```python
from build123d import *

# Parameters (mm, degrees)
SKETCH1_W           = 70
SKETCH1_H           = 70
BOSS_EXTRUDE1_DEPTH = 1
SKETCH2_R           = 25
SKETCH2_R_2         = 23
BOSS_EXTRUDE2_DEPTH = 27
SKETCH3_R           = 2.5
CUT_EXTRUDE1_DEPTH  = 1
SKETCH4_R           = 2.5
CUT_EXTRUDE2_DEPTH  = 1


with BuildPart() as part:
    # Sketch1 → Boss-Extrude1 (new body)
    with BuildSketch(Plane(origin=(0, 0, 0), x_dir=(1, 0, 0), z_dir=(0, 1, 0))):
        Rectangle(SKETCH1_W, SKETCH1_H)
    extrude(amount=BOSS_EXTRUDE1_DEPTH)

    # Sketch2 → Boss-Extrude2 (add)
    with BuildSketch(Plane.XZ):
        with Locations(Location((0, 0, 0), (0, 0, 90))):
            Circle(SKETCH2_R)
        with Locations(Location((0, 0, 0), (0, 0, 270))):
            Circle(SKETCH2_R_2, mode=Mode.SUBTRACT)
    extrude(amount=BOSS_EXTRUDE2_DEPTH)

    # Sketch3 → Cut-Extrude1 (cut)
    with BuildSketch(Plane(origin=(0, 1, 0), x_dir=(1, 0, 0), z_dir=(0, 1, 0))):
        with Locations(Location((0, 0, 0), (0, 0, 270))):
            Circle(SKETCH3_R)
        with Locations(Location((0, 17, 0), (0, 0, 270))):
            Circle(SKETCH3_R)
        with Locations(Location((17, 0, 0), (0, 0, 270))):
            Circle(SKETCH3_R)
        with Locations(Location((0, -17, 0), (0, 0, 270))):
            Circle(SKETCH3_R)
        with Locations(Location((-17, 0, 0), (0, 0, 270))):
            Circle(SKETCH3_R)
    extrude(amount=-CUT_EXTRUDE1_DEPTH, mode=Mode.SUBTRACT)

    # Sketch4 → Cut-Extrude2 (cut)
    with BuildSketch(Plane(origin=(0, 1, 0), x_dir=(1, 0, 0), z_dir=(0, 1, 0))):
        with Locations(Location((21, 21, 0), (0, 0, 270))):
            Circle(SKETCH4_R)
        with Locations(Location((21, -21, 0), (0, 0, 270))):
            Circle(SKETCH4_R)
        with Locations(Location((-21, 21, 0), (0, 0, 270))):
            Circle(SKETCH4_R)
        with Locations(Location((-21, -21, 0), (0, 0, 270))):
            Circle(SKETCH4_R)
    extrude(amount=-CUT_EXTRUDE2_DEPTH, mode=Mode.SUBTRACT)


solid = part.part
```
Build history of the part. All positions in model axes, mm. A direction names the side the tool comes from. Coordinates: 2 decimals unless noted, no trailing zeros. Order: outer loops, then holes, each group sorted by start corner. A loop starts at its lowest first (then second) coordinate and runs counter-clockwise, first axis right, second up.
Item 1: Saw through at D-D on y = -22.5. List the corners of the cut face in (x, z).
Filled in:
outline: circle Ø50 at (0, 0); hole circle Ø46 at (0, 0)
Item 2: Saw through at A-A on x = 0. List the corners of the cut face in (y, z), then the cut area to 3 significant figures.
Filled in:
outline: (-27, -25) - (0, -25) - (0, -35) - (1, -35) - (1, -19.5) - (0, -19.5) - (0, -23) - (-27, -23) - close; (-27, 23) - (0, 23) - (0, 19.5) - (1, 19.5) - (1, 35) - (0, 35) - (0, 25) - (-27, 25) - close; (0, -14.5) - (1, -14.5) - (1, -2.5) - (0, -2.5) - close; (0, 2.5) - (1, 2.5) - (1, 14.5) - (0, 14.5) - close
area: 163 mm2
Item 3: Tool access for faces 4 (the cylindrical face through (19.394, -13.311, -12.365)), 5 (the cylindrical face through (0.1, 0.5, 14.5)): list every direction of +Z, -Z, +X, -X, +Y, -Y with a clear straight run to the whole face (end or side of a thin tool).
Filled in:
face 4: -Y
face 5: +Y, -Y
Item 4: Saw through at C-C on z = -21. List the corners of the cut face in (x, y).
Filled in:
outline: (-35, 0) - (-23.5, 0) - (-23.5, 1) - (-35, 1) - close; (-18.5, 0) - (-13.56, 0) - (-13.56, -27) - (-9.38, -27) - (-9.38, 0) - (9.38, 0) - (9.38, -27) - (13.56, -27) - (13.56, 0) - (18.5, 0) - (18.5, 1) - (-18.5, 1) - close; (23.5, 0) - (35, 0) - (35, 1) - (23.5, 1) - close
Item 5: Mould opens along Z. For faces 1 (the cylindrical face through (22.69, 0.51, -22.84)), 2 (the cylindrical face through (-7.509, -13.311, 23.846)), 3 (the flat face through (22.1, -27, 7.3)) say: released by +Z, released by -Z, zero draft, split by the parting line, or undercut.
Filled in:
face 1: undercut
face 2: split by the parting line
face 3: zero draft
Item 6: Drill centre lines: L1, parallel to X at y = -2, z = 0; L2, parallel to Y at x = -31.5, z = -28; L3, parallel to X at y = -15.5, z = 3. Where is each one in solid material? Low to high.
Filled in:
L1: x = -25 to -23, 23 to 25
L2: y = 0 to 1
L3: x = -24.82 to -22.8, 22.8 to 24.82
Item 7: Saw through at B-B on z = 0. List the corners of the cut face in (x, y), then the cut area to 3 significant figures.
Filled in:
outline: (-35, 0) - (-25, 0) - (-25, -27) - (-23, -27) - (-23, 0) - (-19.5, 0) - (-19.5, 1) - (-35, 1) - close; (-14.5, 0) - (-2.5, 0) - (-2.5, 1) - (-14.5, 1) - close; (2.5, 0) - (14.5, 0) - (14.5, 1) - (2.5, 1) - close; (19.5, 0) - (23, 0) - (23, -27) - (25, -27) - (25, 0) - (35, 0) - (35, 1) - (19.5, 1) - close
area: 163 mm2
Item 8: Drop flat-ended pins along their axis: pin 1 Ø6.5 at (x, z) = (0, 0) entering from -Y; pin 2 Ø1.5 at (x, y) = (-22.5, -10) entering from +Z; pin 3 Ø1 at (x, y) = (16, -3) entering from +Z. Give the stop position or say it passes through.
Filled in:
pin 1: stops at y = 0
pin 2: stops at z = 12.33
pin 3: stops at z = 19.62
